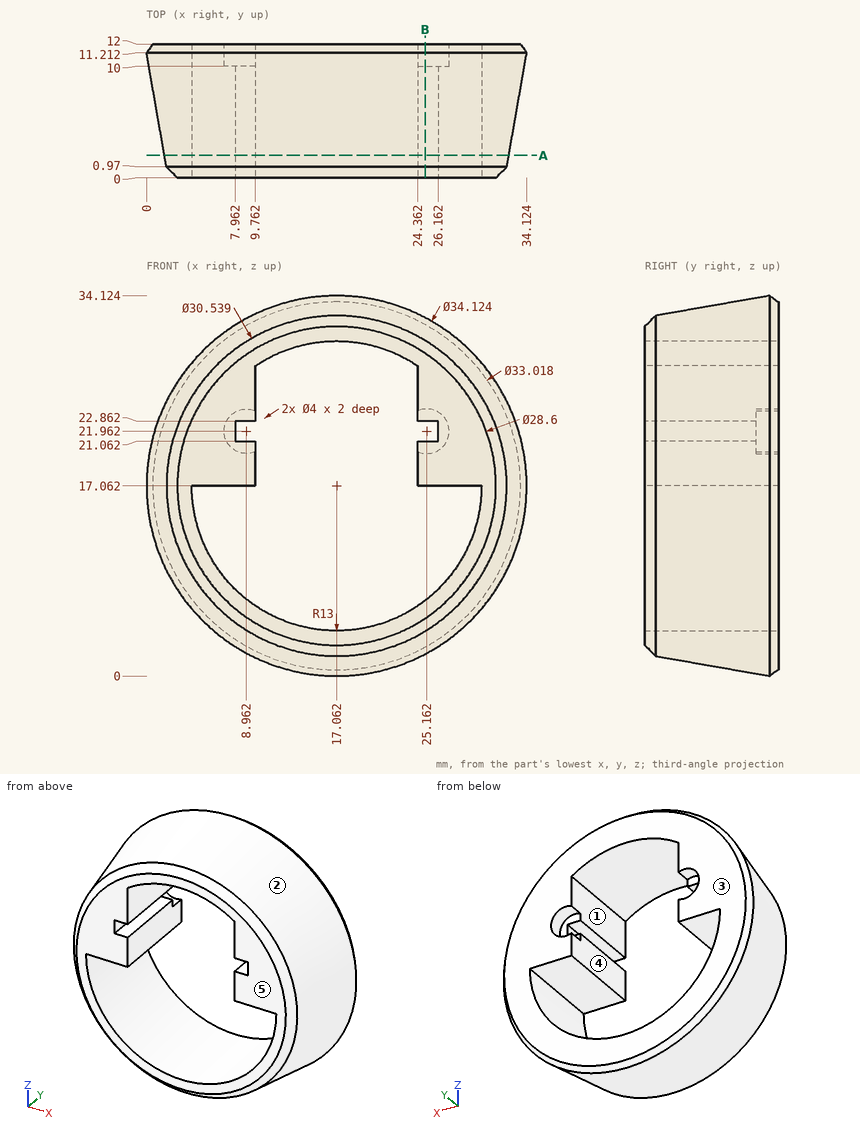
Answer from the drawing. Dimensions are ordinates in mm from the lowest x, y and z of the part. A direction names the side the tool comes from. Give positions to 0.01 mm unless a question says otherwise; leave off trailing zeros. Order: outer loops, then holes, each group sorted by start corner. A loop starts at its lowest first (then second) coordinate and runs counter-clockwise, first axis right, second up. Notation, with made-up numbers: (-36.75, 87) - (-7.75, 87) arc R21 cw to (-7.75, 114) - close; hole circle Ø5 at (51, 28). An arc over 180 degrees is marked (long way). Use one line per item in the form item = value.
1) For the marked faces 4 and 5, determine the directions among +Z, -Z, +X, -X, +Y, -Y from which every point of the face is accessible in a straight line to the end or side of a thin tool.
Verdict:
face_4 = +Y, -Y
face_5 = +Z, -Z, +X, -X, -Y
2) Consider probe 1 along X at (y, z) = (5.5, 25) (1 decimal); probe 2 along X at (y, z) = (7.5, 13) (1 decimal); probe 3 along Y at (x, z) = (10, 4). Determine where each line is inside the solid, lowest interval first. Write a range as [from, to].
Verdict:
probe_1 = [3.1, 9.8], [24.4, 31]
probe_2 = [1.2, 4.7], [29.4, 33]
probe_3 = [0.55, 12]
3) Find section B-B on x = 25. Give the number of separate pieces and of enclosed holes in the cut face, and give its area (3 significant figures).
Verdict:
separate_pieces = 3
enclosed_holes = 0
area = 186 mm^2
4) Find section A-A on y = 2. Determine the outline of the cut face in (x, z).
Verdict:
outline = circle Ø30.9 at (17.06, 17.06); hole (4.06, 17.06) arc R13 ccw to (30.06, 17.06) - (24.36, 17.06) - (24.36, 21.06) - (26.16, 21.06) - (26.16, 22.86) - (24.36, 22.86) - (24.36, 27.82) arc R13 ccw to (9.76, 27.82) - (9.76, 22.86) - (7.96, 22.86) - (7.96, 21.06) - (9.76, 21.06) - (9.76, 17.06) - close
5) Each of these flat-tipped pins is pushed along its axis until it touches: pin 1 (4.5 mm diameter, centred on x = 27, y = 5, fed in from -Z); pin 2 (3 mm diameter, centred on x = 9, z = 21.5, fed in from +Y); pin 3 (1 mm diameter, centred on x = 7.5, y = 3.5, fed in from -Z). Where does it stop, or does it pass through?
Verdict:
pin_1 = 2.98
pin_2 = 10
pin_3 = 4.21
6) The mould has two halves that part along X. Classify the marked faces 1, 2 and 3: released by +X, released by -X, zero draft, split by the parting line, or undercut.
Verdict:
face_1 = undercut
face_2 = split by the parting line
face_3 = zero draft
